Check sheet for the drawn part. Datum: minimum x, y, z corner. Units: mm. Give positions to 0.01 mm unless a question says otherwise; leave off trailing zeros. Write each loop counter-clockwise with the first axis right and the second up, starting at its lowest first coordinate (ties: lowest second). Pieces come first, ordered by that corner, then holes. Notation, with made-up numbers: (54.25, 60.5) -> (106.25, 60.5) arc R12 cw to (106.25, 82.5) -> close; hole circle Ø5 at (-17, 45). An arc over 180 degrees is marked (long way). Answer as CSV lines item,"result". Start each with the question number.
1) Material ranges on L1, parallel to Y at x = 4, z = 0.6; L2, parallel to X at y = 2, z = 1.3, recorded low to high.
2) Gauge pin test, flat end, axial feed: pin 1 Ø1.9 at (x, y) = (34, 4) entering from -Z. Record the tip position at first contact, or that the pin passes through.
3) Sectioned sample at A-A on z = 0.85. Record the cut outline in (x, y), and give its area (3 significant figures).
4) Sectioned sample at B-B on x = 5. Record the cut outline in (y, z).
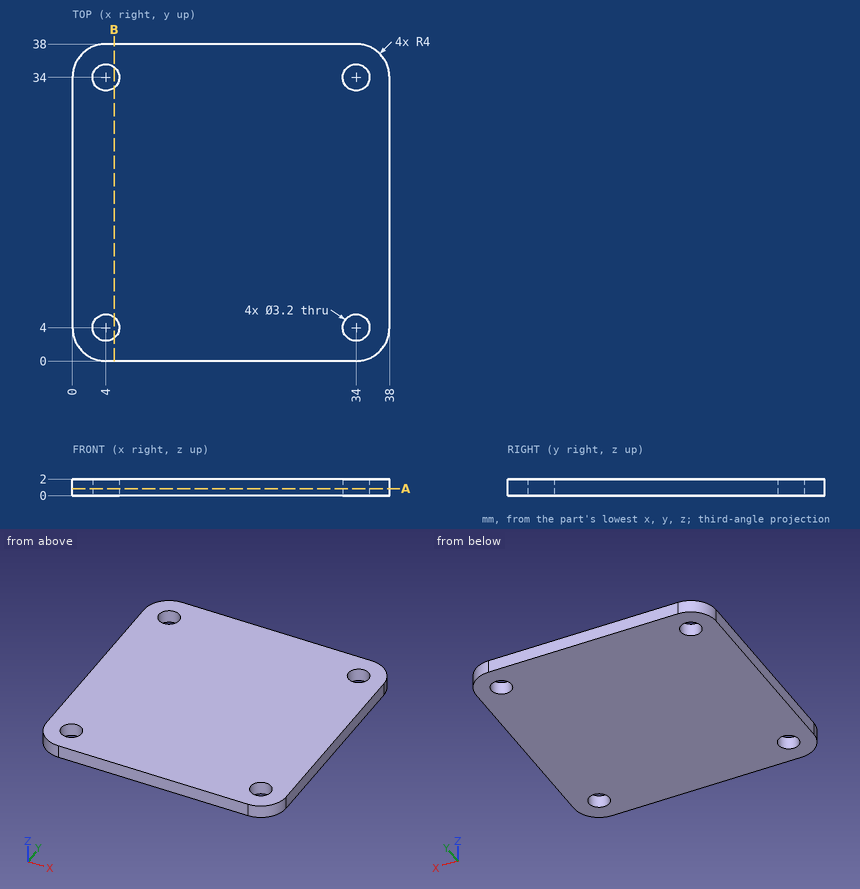
Ans:
1,L1,"y = 0 to 2.4, 5.6 to 32.4, 35.6 to 38"
1,L2,"x = 0.54 to 37.46"
2,pin 1,"passes through"
3,outline,"(0, 4) arc R4 ccw to (4, 0) -> (34, 0) arc R4 ccw to (38, 4) -> (38, 34) arc R4 ccw to (34, 38) -> (4, 38) arc R4 ccw to (0, 34) -> close; hole circle Ø3.2 at (4, 4); hole circle Ø3.2 at (4, 34); hole circle Ø3.2 at (34, 4); hole circle Ø3.2 at (34, 34)"
3,area,"1,400 mm²"
4,outline,"(0, 0) -> (2.75, 0) -> (2.75, 2) -> (0, 2) -> close; (5.25, 0) -> (32.75, 0) -> (32.75, 2) -> (5.25, 2) -> close; (35.25, 0) -> (38, 0) -> (38, 2) -> (35.25, 2) -> close"
